Build history of the part. All positions in model axes, mm. A direction names the side the tool comes from. Give positions to 0.01 mm unless a question says otherwise; leave off trailing zeros. Write each loop counter-clockwise with the first axis right and the second up, starting at its lowest first coordinate (ties: lowest second). Pieces come first, ordered by that corner, then holes. Notation, with made-up numbers: (2, 69.5) -> (39, 69.5) arc R15 cw to (39, 77.5) -> close; hole circle Ø10 at (67, 54). An arc over 180 degrees is marked (long way). Write item = value, one per line. Start each with the question number.
Q1. Drop flat-ended pins along their axis: P1, Ø2.5, axis at x = -22.5, z = -0.5, coming from the -Y side; P2, Ø1.5, axis at y = -1, z = 0.5, coming from the -X side; P3, Ø1, axis at x = -15, y = -1, coming from the +Z side. Give the stop position or say it passes through.
Q2. Saw through at A-A, the plane x = -21. List the corners of the cut face in (y, z).
Q3. Wall check: line 1 (X direction, y = -2.25, z = -1.5); line 2 (Y direction, x = -22.25, z = -2.5); line 3 (Y direction, x = -8.5, z = 0). Give the ranges that are in metal, low to high.
Q4. Saw through at B-B, the plane z = 0. List the corners of the cut face in (x, y), then the cut area to 3 significant figures.
Q5. Tool access for faces 4 (the face through (-19.4, 0, 0)), 5 (the face through (-10.288, 3.905, -0.867)), 6 (the face through (0, 0, 0)): list every direction of +Z, -Z, +X, -X, +Y, -Y with a clear straight run to the whole face (end or side of a thin tool).
Q6. Saw through at C-C, the plane x = -13.75. List the corners of the cut face in (y, z).
Q7. Mould opens along Y. For faces 1 (the face through (-20.244, -4.186, -0.55)), 2 (the face through (-24.4, -0.1, 3.2)), 3 (the face through (-21.935, 1.233, 2.175)) say: pulls with the +Y half, pulls with the -Y half, needs draft (parallel to the pull), parting line crosses it, or undercut.
from build123d import *

# Parameters (mm, degrees)
KES_EKSTR_ZYON1_DEPTH = 5
RADYUS2_R             = 0.3


with BuildPart() as part:
    # Çizim1 → Döndür1 (revolve)
    with BuildSketch(Plane.XY, mode=Mode.PRIVATE) as d_nd_r1_sk:
        Polygon((0, 0), (0, 4), (-20, 4), (-24.4, 8), (-24.4, 0), align=None)
    revolve(d_nd_r1_sk.sketch.rotate(Axis((-24.4, 0, 0), (1, 0, 0)), 90), axis=Axis((-24.4, 0, 0), (1, 0, 0)))

    # Çizim2 → Kes-Ekstrüzyon1 (cut)
    with BuildSketch(Plane.ZY.offset(24.4)):
        Polygon((2.886751346, 0), (1.443375673, 2.5), (-1.443375673, 2.5), (-2.886751346, 0), (-1.443375673, -2.5), (1.443375673, -2.5), align=None)
    extrude(amount=-KES_EKSTR_ZYON1_DEPTH, mode=Mode.SUBTRACT)

    # Radyus2
    radyus2_edges = [part.edges().sort_by_distance(p)[0] for p in [
        (-24.4, 0, -8),
        (0, 0, -4),
    ]]
    fillet(radyus2_edges, radius=RADYUS2_R)


solid = part.part
Report:
q1.P1 = -7.39
q1.P2 = -19.4
q1.P3 = 3.97
q2.outline = circle Ø9.82 at (0, 0); hole (-2.5, -1.44) -> (0, -2.89) -> (2.5, -1.44) -> (2.5, 1.44) -> (0, 2.89) -> (-2.5, 1.44) -> close
q3.line_1 = -19.4 to 0
q3.line_2 = -5.5 to -0.67, 0.67 to 5.5
q3.line_3 = -4 to 4
q4.outline = (-24.4, -7.32) arc R0.3 ccw to (-23.9, -7.54) -> (-20, -4) -> (-0.3, -4) arc R0.3 ccw to (0, -3.7) -> (0, 3.7) arc R0.3 ccw to (-0.3, 4) -> (-20, 4) -> (-23.9, 7.54) arc R0.3 ccw to (-24.4, 7.32) -> (-24.4, 2.5) -> (-19.4, 2.5) -> (-19.4, -2.5) -> (-24.4, -2.5) -> close
q4.area = 188 mm2
q5.face_4 = -X
q5.face_5 = +X
q5.face_6 = +Z, -Z, +X, +Y, -Y
q6.outline = circle Ø8 at (0, 0)
q7.face_1 = parting line crosses it
q7.face_2 = needs draft
q7.face_3 = undercut
